Geometry check sheet. Reference: the model listing, model coordinates, mm. Round coordinates to 2 decimals unless told otherwise and drop trailing zeros. Loops run counter-clockwise (first coordinate to the right, second up) from the corner with the lowest first, then second, coordinate; pieces in that order, holes last. Notation, with made-up numbers: (59, 84.25) - (71, 84.25) arc R10 ccw to (71, 98.25) - close; hole circle Ø2 at (47.5, 69.5). An arc over 180 degrees is marked (long way). Answer as CSV lines item,"result". Start each with the question number.
1) Cross-section at B-B on y = 8. Record the boundary of the cut face in (x, z) (3 decimals), and give its area (3 significant figures).
2) Cross-section at C-C on z = 6.75. Record the boundary of the cut face in (x, y) (3 decimals).
3) Depth check by flat-ended pin: P1, Ø6, axis at x = -38.1, y = 9.525, coming from the -Z side; P2, Ø10, axis at x = -20, y = 18, coming from the -Z side. Enter the tip coordinate at first touch or a pass-through.
4) Draft check along X on faces 1 (the flat face through (-63.5, 12, 5)), 2 (the flat face through (63.5, 12, 5)), 3 (the cylindrical face through (7.067, 10.357, 4.696)). Enter one of: released by +X, released by -X, zero draft, split by the parting line, or undercut.
5) Thickness scan on line 1 along X through (y, z) = (13.25, 6); line 2 along Y through (x, z) = (-38.1, 3) (3 decimals); line 3 along X through (y, z) = (13.5, 5.5). Record the ranges inside material, lowest first.
6) Cross-section at A-A on x = -38.1. Record the boundary of the cut face in (y, z) (3 decimals), and give its area (3 significant figures).
from build123d import *

# Parameters (mm, degrees)
SKETCH1_W           = 127
SKETCH1_H           = 44.45
BOSS_EXTRUDE1_DEPTH = 9.525
SKETCH6_R           = 4.8
CUT_EXTRUDE1_DEPTH  = 68.947967225
SKETCH10_R          = 2.286
CUT_EXTRUDE2_DEPTH  = 3.81
SKETCH13_W          = 127
SKETCH13_H          = 49.203053771
CUT_EXTRUDE3_DEPTH  = 68.947967225
SKETCH15_R          = 5.652121823
CUT_EXTRUDE4_DEPTH  = 68.947967225


with BuildPart() as part:
    # Sketch1 → Boss-Extrude1 (new body)
    with BuildSketch(Plane.XY):
        Rectangle(SKETCH1_W, SKETCH1_H)
    extrude(amount=BOSS_EXTRUDE1_DEPTH)

    # Sketch6 → Cut-Extrude1 (cut, through all)
    with BuildSketch(Plane.XY):
        with Locations(Location((-38.1, 9.525, 0), (0, 0, 180))):
            Circle(SKETCH6_R)
    extrude(amount=CUT_EXTRUDE1_DEPTH, mode=Mode.SUBTRACT)

    # Sketch10 → Cut-Extrude2 (cut)
    with BuildSketch(Plane.XY.offset(9.525)):
        with Locations((-46.11545283, -16.764)):
            Circle(SKETCH10_R)
    extrude(amount=-CUT_EXTRUDE2_DEPTH, mode=Mode.SUBTRACT)

    # Sketch13 → Cut-Extrude3 (cut, through all)
    with BuildSketch(Plane(origin=(0, 0, 0), x_dir=(-1, 0, 0), z_dir=(0, 0, -1))):
        with Locations((0, -22.225000001)):
            Rectangle(SKETCH13_W, SKETCH13_H)
    extrude(amount=-CUT_EXTRUDE3_DEPTH, mode=Mode.SUBTRACT)

    # Sketch15 → Cut-Extrude4 (cut, through all)
    with BuildSketch(Plane(origin=(0, 0, 0), x_dir=(-1, 0, 0), z_dir=(0, 0, -1))):
        with Locations((-5.842, 15.875)):
            Circle(SKETCH15_R)
    extrude(amount=-CUT_EXTRUDE4_DEPTH, mode=Mode.SUBTRACT)


solid = part.part
Answer block:
1,outline,"(-63.5, 0) - (-42.651, 0) - (-42.651, 9.525) - (-63.5, 9.525) - close; (-33.549, 0) - (63.5, 0) - (63.5, 9.525) - (-33.549, 9.525) - close"
1,area,"1,120 mm^2"
2,outline,"(-63.5, 2.377) - (63.5, 2.377) - (63.5, 22.225) - (-63.5, 22.225) - close; hole circle Ø9.6 at (-38.1, 9.525); hole circle Ø11.304 at (5.842, 15.875)"
3,P1,"passes through"
3,P2,"stops at z = 0"
4,face 1,"released by -X"
4,face 2,"released by +X"
4,face 3,"undercut"
5,line 1,"x = -63.5 to -41.13, -35.07 to 0.84, 10.85 to 63.5"
5,line 2,"y = 2.377 to 4.725, 14.325 to 22.225"
5,line 3,"x = -63.5 to -40.79, -35.41 to 0.71, 10.97 to 63.5"
6,outline,"(2.377, 0) - (4.725, 0) - (4.725, 9.525) - (2.377, 9.525) - close; (14.325, 0) - (22.225, 0) - (22.225, 9.525) - (14.325, 9.525) - close"
6,area,"97.6 mm^2"
